The listing builds one solid part. Answer for the finished solid, in the listing's coordinates (mm). A direction names the side the tool comes from. Coordinates: 2 decimals unless noted, no trailing zeros. Loops run counter-clockwise (first coordinate to the right, second up) from the corner with the lowest first, then second, coordinate; pieces in that order, holes last. Notation, with made-up numbers: (69, 68.25) -> (99, 68.25) arc R26 cw to (99, 100.25) -> close; hole circle Ø11 at (-14, 48). An arc over 180 degrees is marked (long way). Answer in a Markdown table with one row per item.
```python
from build123d import *

# Parameters (mm, degrees)
SKETCH1_W                      = 19.5
SKETCH1_H                      = 10.2
BOSS_EXTRUDE1_DEPTH            = 5.8
SKETCH4_W                      = 0.5
SKETCH4_H                      = 2.8
BOSS_EXTRUDE4_DEPTH            = 3.2
SKETCH5_W                      = 0.5
SKETCH5_H                      = 2.8
BOSS_EXTRUDE5_DEPTH            = 3.2
SKETCH6_W                      = 0.5
SKETCH6_H                      = 2.8
BOSS_EXTRUDE6_DEPTH            = 3.2
F_2_5_2_5_DIAMETER_HOLE1_D     = 2.5
F_2_5_2_5_DIAMETER_HOLE1_DEPTH = 10
F_2_5_2_5_DIAMETER_HOLE1_TIP   = 0.751075774
BOSS_EXTRUDE7_DEPTH            = 3


with BuildPart() as part:
    # Sketch1 → Boss-Extrude1 (new body)
    with BuildSketch(Plane.XY.offset(5)):
        with Locations((-9.915879305, -7.543983402)):
            Rectangle(SKETCH1_W, SKETCH1_H)
    extrude(amount=-BOSS_EXTRUDE1_DEPTH)

    # Sketch4 → Boss-Extrude4 (add)
    with BuildSketch(Plane.XZ.offset(12.643983402)):
        with Locations((-9.665879305, 3.25)):
            Rectangle(SKETCH4_W, SKETCH4_H)
    extrude(amount=BOSS_EXTRUDE4_DEPTH)

    # Sketch5 → Boss-Extrude5 (add)
    with BuildSketch(Plane.XZ.offset(12.643983402)):
        with Locations((-17.165879305, 3.25)):
            Rectangle(SKETCH5_W, SKETCH5_H)
    extrude(amount=BOSS_EXTRUDE5_DEPTH)

    # Sketch6 → Boss-Extrude6 (add)
    with BuildSketch(Plane.XZ.offset(12.643983402)):
        with Locations((-2.165879305, 3.25)):
            Rectangle(SKETCH6_W, SKETCH6_H)
    extrude(amount=BOSS_EXTRUDE6_DEPTH)

    # Ø2.5 (2.5) Diameter Hole1
    with Locations(Plane(origin=(0, 0, -0.8), x_dir=(-1, 0, 0), z_dir=(0, 0, -1))):
        with Locations((14.665879305, -9.443983402), (5.165879305, -9.443983402)):
            Hole(F_2_5_2_5_DIAMETER_HOLE1_D / 2, depth=F_2_5_2_5_DIAMETER_HOLE1_DEPTH)
            with Locations((0, 0, -(F_2_5_2_5_DIAMETER_HOLE1_DEPTH + F_2_5_2_5_DIAMETER_HOLE1_TIP / 2))):  # 118° drill point
                Cone(0, F_2_5_2_5_DIAMETER_HOLE1_D / 2, F_2_5_2_5_DIAMETER_HOLE1_TIP, mode=Mode.SUBTRACT)

    # Sketch9 → Boss-Extrude7 (add)
    with BuildSketch(Plane.XY):
        Polygon((-2.965879305, -1.193983402), (-2.965879305, -2.443983402), (-3.265879305, -2.443983402), (-3.265879305, -1.455557189), (-21.532448725, 1.056016598), (-21.491584492, 1.353220424), align=None)
    extrude(amount=BOSS_EXTRUDE7_DEPTH)


solid = part.part
```
Item 1: A cutting plane is placed at A-A, the plane y = -9.75. Determine the outline of the cut face in (x, z), plus the area to 3 significant figures.
Findings below:
| item | result |
|---|---|
| outline | (-19.67, -0.8) -> (-15.88, -0.8) -> (-15.88, 5) -> (-19.67, 5) -> close; (-13.45, -0.8) -> (-6.38, -0.8) -> (-6.38, 5) -> (-13.45, 5) -> close; (-3.95, -0.8) -> (-0.17, -0.8) -> (-0.17, 5) -> (-3.95, 5) -> close |
| area | 85.0 mm2 |
Item 2: A cutting plane is placed at B-B, the plane z = 4.2. Determine the outline of the cut face in (x, y), plus the area to 3 significant figures.
Findings below:
| item | result |
|---|---|
| outline | (-19.67, -12.64) -> (-17.42, -12.64) -> (-17.42, -15.84) -> (-16.92, -15.84) -> (-16.92, -12.64) -> (-9.92, -12.64) -> (-9.92, -15.84) -> (-9.42, -15.84) -> (-9.42, -12.64) -> (-2.42, -12.64) -> (-2.42, -15.84) -> (-1.92, -15.84) -> (-1.92, -12.64) -> (-0.17, -12.64) -> (-0.17, -2.44) -> (-19.67, -2.44) -> close; hole circle Ø2.5 at (-14.67, -9.44); hole circle Ø2.5 at (-5.17, -9.44) |
| area | 194 mm2 |
Item 3: A tool of negligible diameter and unlimited length cuts with its end or side. For faces 4 (the face through (-2.966, -2, 1)), 5 (the face through (-17.416, -14, 3)), 6 (the face through (-1.916, -14, 3)), 7 (the face through (-2.416, -14, 3)), 8 (the face through (-12.271, -0.217, 1.479)), from which of +Z, -Z, +X, -X, +Y, -Y can it reach the whole face along a straight path? Write none if from no direction.
Findings below:
| item | result |
|---|---|
| face 4 | +Z, -Z, +X, +Y |
| face 5 | +Z, -Z, -X, -Y |
| face 6 | +Z, -Z, +X, -Y |
| face 7 | +Z, -Z, -Y |
| face 8 | +Z, -Z, -X |
Item 4: Flat-ended cylindrical pins translate along their axes: pin 1 Ø0.8 at (y, z) = (-14, 4) entering from -X; pin 2 Ø2 at (y, z) = (-9, 2.5) entering from -X; pin 3 Ø1.9 at (x, y) = (-12, -1) entering from +Z; pin 4 Ø8 at (x, y) = (-3, -2) entering from -Z. Find the tip coordinate at first contact, or state that the pin passes through.
Findings below:
| item | result |
|---|---|
| pin 1 | stops at x = -17.42 |
| pin 2 | stops at x = -19.67 |
| pin 3 | stops at z = 3 |
| pin 4 | stops at z = -0.8 |
Item 5: Find the intervals of material crossed by probe 1 along X at (y, z) = (-14.5, 3.9); probe 2 along Y at (x, z) = (-15.75, 2.85); probe 3 along X at (y, z) = (-4, 0.85), in increasing order.
Findings below:
| item | result |
|---|---|
| probe 1 | x = -17.42 to -16.92, -9.92 to -9.42, -2.42 to -1.92 |
| probe 2 | y = -12.64 to -10.07, -8.82 to -2.44, 0.26 to 0.56 |
| probe 3 | x = -19.67 to -0.17 |
Item 6: A cutting plane is placed at C-C, the plane x = -14.25. Determine the outline of the cut face in (y, z), plus the area to 3 significant figures.
Findings below:
| item | result |
|---|---|
| outline | (-12.64, -0.8) -> (-10.62, -0.8) -> (-10.62, 5) -> (-12.64, 5) -> close; (-8.27, -0.8) -> (-2.44, -0.8) -> (-2.44, 5) -> (-8.27, 5) -> close; (0.05, 0) -> (0.36, 0) -> (0.36, 3) -> (0.05, 3) -> close |
| area | 46.4 mm2 |
Item 7: Determine the mould class of faces 1 (the face through (-3.266, -2, 1)), 2 (the face through (-9.916, -14, 3)), 3 (the face through (-0.166, -8, 2)) for opening direction X: +X half, -X half, draft (parallel to the pull), parting line (faces both ways), or undercut.
Findings below:
| item | result |
|---|---|
| face 1 | -X half |
| face 2 | undercut |
| face 3 | +X half |
Item 8: A cutting plane is placed at D-D, the plane x = -11.5. Determine the outline of the cut face in (y, z).
Findings below:
| item | result |
|---|---|
| outline | (-12.64, -0.8) -> (-2.44, -0.8) -> (-2.44, 5) -> (-12.64, 5) -> close; (-0.32, 0) -> (-0.02, 0) -> (-0.02, 3) -> (-0.32, 3) -> close |
